Build history of the part. All positions in model axes, mm. Face numbers are marked on the shaded views. A direction names the side the tool comes from. Coordinates: 2 decimals unless noted, no trailing zeros. Loops run counter-clockwise (first coordinate to the right, second up) from the corner with the lowest first, then second, coordinate; pieces in that order, holes last.
Item 1: Cut at B-B (y = 12). List the corners of the cut face in (x, z).
Item 2: Cut at A-A (x = 40.5). List the corners of the cut face in (y, z).
Item 3: Mould opens along Z. For the marked faces 5, 6, 7 and 8 say: released by +Z, released by -Z, zero draft, split by the parting line, or undercut.
Item 4: Cut at C-C (y = -21.5). List the corners of the cut face in (x, z), and give its area (3 significant figures).
Item 5: Drill centre lines: line 1 along Y through (x, z) = (3.5, 3.5); line 2 along Y through (x, z) = (51.5, 12.25); line 3 along Z through (x, y) = (9, 13). Where is each one in solid material? Low to high.
Item 6: 3-axis set-ups, long thin cutter, end or side, ignore diameter. For the marked faces 1, 2, 3 and 4: which of +Z, -Z, +X, -X, +Y, -Y reach the whole face in a straight line?
Item 7: Flat gauge pins, fed straight in: pin 1 (3.5 mm diameter, centred on x = 23.5, y = -22, fed in from -Z); pin 2 (5 mm diameter, centred on x = 66, z = -2.5, fed in from -Y); pin 3 (10 mm diameter, centred on x = 53.5, y = -22, fed in from +Z). Where does each tip first touch, or does it go through?
Item 8: Cut at D-D (x = 28). List the corners of the cut face in (y, z).
from build123d import *

# Parameters (mm, degrees)
F1_DEPTH      = 75
F2_W          = 3.3
F2_H          = 5
F3_DEPTH      = 75
F5_DEPTH      = 3
F6_ANGLE      = -30
F7_W          = 15
F7_H          = 8
F8_DEPTH      = 75
F9_R          = 5
F10_T1_DEPTH  = 75
F10_T6_DEPTH  = 82.2168783649
F10_T11_DEPTH = 82.2168783649
F10_T17_DEPTH = 89.4337567297
F10_T23_DEPTH = 82.2168783649
F10_T25_DEPTH = 100
F11_R         = 30


# Not quite as in the source:
# - a fillet or chamfer that OpenCascade refuses, or shapes differently, is made with other operations: its cross-section is extruded or revolved along the edge and cut away or added


with BuildPart() as f1:
    # F0 (on Right) → F1 (new body)
    with BuildSketch(Plane.YZ):
        Polygon((3, 13.5), (0, 13.5), (0, -13), (3, -13), (3, 8.5), (10, 8.5), (10, 0), (17.5, 0), (17.5, 13.5), (10, 13.5), align=None)
    extrude(amount=F1_DEPTH)

    # F4 (on Front) → F5 (cut, through all)
    with BuildSketch(Plane.XZ):
        Polygon((11.5, 2.5), (11.5, -7.5), (13, -7.5), (11.1212156062, -13), (33, -13), (33, -7.4999375637), (33, 2.5), align=None)
        Polygon((63.5, 2.5), (42, 2.5), (42, -7.4999375637), (42, -13), (64.044855535, -13), (62, -7.5), (63.5, -7.5), align=None)
    extrude(amount=-F5_DEPTH, mode=Mode.SUBTRACT)


with BuildPart() as f3:
    # F2 (on Right) → F3 (new body)
    with BuildSketch(Plane.YZ):
        Polygon((-23.3, 13.5), (-28.3, 13.5), (-28.3, 0.5), (-23.3, 0.5), (-23.3, 8.5), align=None)
        with Locations((-21.65, 11)):
            Rectangle(F2_W, F2_H)
        Polygon((-15, 13.5), (-20, 13.5), (-20, 8.5), (-20, -6.5), (-15, -6.5), align=None)
    extrude(amount=F3_DEPTH)


with BuildPart() as f1_1:
    # F6: moved
    add(f1.part.rotate(Axis((37.5, 0, 13.5), (-1, 0, 0)), F6_ANGLE))


    add(f3.part)  # F8 merges F3
    # F7 (on Right) → F8 (join)
    with BuildSketch(Plane.YZ):
        with Locations((-7.5, 9.5)):
            Rectangle(F7_W, F7_H)
        Polygon((5.764299538, 5.5), (0, 13.5), (0, 5.5), align=None)
    extrude(amount=F8_DEPTH)

    # F9
    f9_edges = [f1_1.edges().sort_by_distance(p)[0] for p in [
        (37.5, 15.155445, 22.25),
    ]]
    fillet(f9_edges, radius=F9_R)

    # F10: fillet of radius 5 on 3 edges, made by hand

    # F10_s2 → F10_t1 (join)
    with BuildSketch(Plane.YZ):
        with BuildLine():
            ThreePointArc((-10, 5.5), (-13.5355339059, 4.0355339059), (-15, 0.5))
            Line((-15, 0.5), (-15, 5.5))
            Line((-15, 5.5), (-10, 5.5))
        make_face()
    extrude(amount=F10_T1_DEPTH)


with BuildPart() as f10_tool4:
    # F10_s5 → F10_t6 (new body)
    with BuildSketch(Plane.YZ):
        with BuildLine():
            ThreePointArc((6.0621778265, 3), (4.2320508076, 4.8301270189), (1.7320508076, 5.5))
            Line((1.7320508076, 5.5), (4.6188021535, 5.5))
            Line((4.6188021535, 5.5), (6.0621778265, 3))
        make_face()
    extrude(amount=F10_T6_DEPTH)

    split(bisect_by=Plane.YZ.offset(11.5), keep=Keep.BOTTOM)


with BuildPart() as f1_2:
    add(f1_1.part)

    # F10_t3: union F10_tool4
    add(f10_tool4.part)


with BuildPart() as f10_tool9:
    # F10_s10 → F10_t11 (new body)
    with BuildSketch(Plane.YZ.offset(-7.2168783649)):
        with BuildLine():
            ThreePointArc((6.0621778265, 3), (4.2320508076, 4.8301270189), (1.7320508076, 5.5))
            Line((1.7320508076, 5.5), (4.6188021535, 5.5))
            Line((4.6188021535, 5.5), (6.0621778265, 3))
        make_face()
    extrude(amount=F10_T11_DEPTH)

    split(bisect_by=Plane(origin=(0, -0.3456714755, 0.5987205584), x_dir=(1, 0, 0), z_dir=(0, -0.5, 0.8660254038)), keep=Keep.TOP)

    split(bisect_by=Plane.YZ.offset(11.5), keep=Keep.TOP)


with BuildPart() as f1_3:
    add(f1_2.part)

    # F10_t8: union F10_tool9
    add(f10_tool9.part)


with BuildPart() as f10_tool15:
    # F10_s16 → F10_t17 (new body)
    with BuildSketch(Plane.YZ.offset(-7.2168783649)):
        with BuildLine():
            ThreePointArc((6.0621778265, 3), (4.2320508076, 4.8301270189), (1.7320508076, 5.5))
            Line((1.7320508076, 5.5), (4.6188021535, 5.5))
            Line((4.6188021535, 5.5), (6.0621778265, 3))
        make_face()
    extrude(amount=F10_T17_DEPTH)

    split(bisect_by=Plane.YZ.offset(42), keep=Keep.BOTTOM)

    split(bisect_by=Plane.YZ.offset(33), keep=Keep.TOP)


with BuildPart() as f1_4:
    add(f1_3.part)

    # F10_t14: union F10_tool15
    add(f10_tool15.part)


with BuildPart() as f10_tool21:
    # F10_s22 → F10_t23 (new body)
    with BuildSketch(Plane.YZ.offset(-7.2168783649)):
        with BuildLine():
            ThreePointArc((6.0621778265, 3), (4.2320508076, 4.8301270189), (1.7320508076, 5.5))
            Line((1.7320508076, 5.5), (4.6188021535, 5.5))
            Line((4.6188021535, 5.5), (6.0621778265, 3))
        make_face()
    extrude(amount=F10_T23_DEPTH)

    split(bisect_by=Plane.YZ.offset(63.5), keep=Keep.TOP)


with BuildPart() as f1_5:
    add(f1_4.part)

    # F10_t20: union F10_tool21
    add(f10_tool21.part)

    # F10_s26 → F10_t25 (cut)
    with BuildSketch(Plane.YZ.offset(-12.5)):
        with BuildLine():
            ThreePointArc((-15, -1.5), (-16.4644660941, -5.0355339059), (-20, -6.5))
            Line((-20, -6.5), (-15, -6.5))
            Line((-15, -6.5), (-15, -1.5))
        make_face()
    extrude(amount=F10_T25_DEPTH, mode=Mode.SUBTRACT)

    # F11
    f11_edges = [f1_5.edges().sort_by_distance(p)[0] for p in [
        (37.5, 0, 13.5),
    ]]
    fillet(f11_edges, radius=F11_R)


solid = f1_5.part
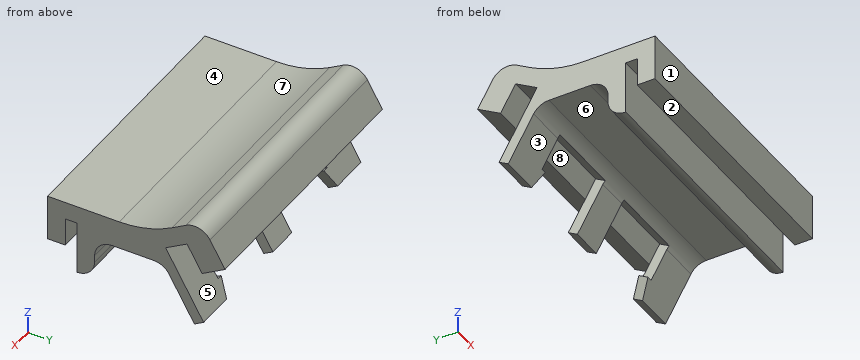
Filled sheet:
1. outline: (0, -7.28) - (11.98, -7.28) - (13, -3.82) - (11.5, -3.82) - (11.5, -1.28) - (0, -1.28) - close; (0, 12.72) - (75, 12.72) - (75, 20.24) - (0, 20.24) - close; (33, -7.28) - (42, -7.28) - (42, -1.28) - (33, -1.28) - close; (62, -3.82) - (63.12, -7.28) - (75, -7.28) - (75, -1.28) - (63.5, -1.28) - (63.5, -3.82) - close
2. outline: (-28.3, 0.5) - (-23.3, 0.5) - (-23.3, 8.5) - (-20, 8.5) - (-20, -6.5) arc R5 ccw to (-15, -1.5) - (-15, 0.5) arc R5 cw to (-10, 5.5) - (1.73, 5.5) arc R5 cw to (6.06, 3) - (13.25, -9.45) - (15.85, -7.95) - (5.1, 10.67) - (11.16, 14.17) - (15.41, 6.81) - (21.91, 10.56) - (17.66, 17.92) arc R5 ccw to (10.83, 19.75) - (6.96, 17.52) arc R30 cw to (-8.04, 13.5) - (-28.3, 13.5) - close
3. face 5: undercut
3. face 6: released by -Z
3. face 7: released by +Z
3. face 8: undercut
4. outline: (0, 8.5) - (75, 8.5) - (75, 13.5) - (0, 13.5) - close
4. area: 375 mm2
5. line 1: y = -28.3 to -23.3, -20 to -14, 5.73 to 9.24
5. line 2: y = -28.3 to 7.83, 12.27 to 20.93
5. line 3: z = -9.02 to -3.02, 10.98 to 20.41
6. face 1: +Z, -Z, +X, -X, -Y
6. face 2: -Z, +X, -X, -Y
6. face 3: -Z, +X, -X
6. face 4: +Z, +X, -X, -Y
7. pin 1: stops at z = 0.5
7. pin 2: stops at y = -20
7. pin 3: stops at z = 13.5
8. outline: (-28.3, 0.5) - (-23.3, 0.5) - (-23.3, 8.5) - (-20, 8.5) - (-20, -6.5) arc R5 ccw to (-15, -1.5) - (-15, 0.5) arc R5 cw to (-10, 5.5) - (1.73, 5.5) arc R5 cw to (5.39, 3.91) - (8.1, 5.47) - (5.1, 10.67) - (11.16, 14.17) - (15.41, 6.81) - (21.91, 10.56) - (17.66, 17.92) arc R5 ccw to (10.83, 19.75) - (6.96, 17.52) arc R30 cw to (-8.04, 13.5) - (-28.3, 13.5) - close
